Part model, mm, in its own coordinate system. Give positions to 0.01 mm unless a question says otherwise; leave off trailing zeros. Order: outer loops, then holes, each group sorted by start corner. A loop starts at its lowest first (then second) coordinate and runs counter-clockwise, first axis right, second up.
from build123d import *

# Parameters (mm, degrees)
F1_DEPTH = 4.7625


# Not quite as in the source:
# - a length typed as a fraction of an inch, garbled in the dataset ("3 / 203.2 mm" for 3/8 in), is restored


with BuildPart() as f1:
    # F0 (on Front) → F1 (new body)
    with BuildSketch(Plane.XZ):
        Polygon((342.7002896502, -163.4048530862), (380.145872664, 138.4910887061), (-377.0557005115, 138.4910887061), (-345.7904618027, -113.577324326), align=None)
    extrude(amount=F1_DEPTH)


with BuildPart() as f2_1:
    # F2: instance of F1
    add(f1.part.mirror(Plane.YZ))


solid = f2_1.part
Item 1: Pull direction X, two halves, no side cores. Call faces 1 (the face through (6.365, -2.348, -138.142)), 2 (the face through (-361.16, -2.35, -14.57)), 3 (the face through (4, -4.762, -10)): released by +X, released by -X, zero draft, split by the parting line, or undercut.
Item 2: Band-saw the part on A-A on y = -2.05. List the corners of the cut face in (x, z), plus the area to 3 significant figures.
Item 3: Drill centre lines: probe 1 along Z at (x, y) = (-210, -3.4); probe 2 along X at (y, z) = (-3.1, 4.5); probe 3 along X at (y, z) = (-2.65, -76). Where is each one in solid material? Low to high.
Item 4: Band-saw the part on B-B on z = -2. List the corners of the cut face in (x, y).
Working result:
1. face 1: released by +X
1. face 2: released by -X
1. face 3: zero draft
2. outline: (-380.15, 138.49) - (-342.7, -163.4) - (345.79, -113.58) - (377.06, 138.49) - close
2. area: 200,000 mm2
3. probe 1: z = -153.8 to 138.49
3. probe 2: x = -363.53 to 360.44
3. probe 3: x = -353.54 to 350.45
4. outline: (-362.72, -4.76) - (359.63, -4.76) - (359.63, 0) - (-362.72, 0) - close
